Work out the finished part from the listing and answer in its coordinate system (mm). Round coordinates to 2 decimals unless told otherwise and drop trailing zeros. Loops run counter-clockwise (first coordinate to the right, second up) from the corner with the lowest first, then second, coordinate; pieces in that order, holes last. Notation, with made-up numbers: (18, 20) - (69, 20) arc R30 ccw to (69, 43) - close; hole circle Ø1 at (-16, 64). An arc over 180 degrees is marked (long way). Return JSON: item names as keys, results as strings.
from build123d import *

# Parameters (mm, degrees)
SKETCH2_R           = 4
BOSS_EXTRUDE1_DEPTH = 5
FILLET1_R           = 40


with BuildPart() as part:
    # Sketch2 → Boss-Extrude1 (new body)
    with BuildSketch(Plane(origin=(0, -112.700994014, 0), x_dir=(1, 0, 0), z_dir=(0, 1, 0))):
        Polygon((271.436244825, 21.453222376), (186.436244825, 21.453222376), (186.436244825, 274.737493623), (-183.563755175, 274.737493623), (-183.563755175, 21.453222376), (-268.563755175, 21.453222376), (-268.563755175, -91.978235129), (-183.563755175, -91.978235129), (-183.563755175, -345.262506377), (186.436244825, -345.262506377), (186.436244825, -91.978235129), (271.436244825, -91.978235129), align=None)
        with Locations(Location((156.436244825, -325.262506377, 0), (0, 0, 270))):
            Circle(SKETCH2_R, mode=Mode.SUBTRACT)
        with Locations(Location((126.436244825, -325.262506377, 0), (0, 0, 270))):
            Circle(SKETCH2_R, mode=Mode.SUBTRACT)
        with Locations(Location((251.436244825, -61.978235129, 0), (0, 0, 270))):
            Circle(SKETCH2_R, mode=Mode.SUBTRACT)
        with Locations(Location((-153.563755175, -325.262506377, 0), (0, 0, 270))):
            Circle(SKETCH2_R, mode=Mode.SUBTRACT)
        with Locations(Location((-123.563755175, -325.262506377, 0), (0, 0, 270))):
            Circle(SKETCH2_R, mode=Mode.SUBTRACT)
        with Locations(Location((-248.563755175, -61.978235129, 0), (0, 0, 270))):
            Circle(SKETCH2_R, mode=Mode.SUBTRACT)
        with Locations(Location((51.436244825, -275.262506377, 0), (0, 0, 270))):
            Circle(SKETCH2_R, mode=Mode.SUBTRACT)
        with Locations(Location((51.436244825, -65.262506377, 0), (0, 0, 270))):
            Circle(SKETCH2_R, mode=Mode.SUBTRACT)
        with Locations(Location((51.436244825, -5.262506377, 0), (0, 0, 90))):
            Circle(SKETCH2_R, mode=Mode.SUBTRACT)
        with Locations(Location((51.436244825, 204.737493623, 0), (0, 0, 90))):
            Circle(SKETCH2_R, mode=Mode.SUBTRACT)
        with Locations(Location((-248.563755175, -8.546777624, 0), (0, 0, 90))):
            Circle(SKETCH2_R, mode=Mode.SUBTRACT)
        with Locations(Location((-123.563755175, 254.737493623, 0), (0, 0, 90))):
            Circle(SKETCH2_R, mode=Mode.SUBTRACT)
        with Locations(Location((-153.563755175, 254.737493623, 0), (0, 0, 90))):
            Circle(SKETCH2_R, mode=Mode.SUBTRACT)
        with Locations(Location((126.436244825, 254.737493623, 0), (0, 0, 90))):
            Circle(SKETCH2_R, mode=Mode.SUBTRACT)
        with Locations(Location((156.436244825, 254.737493623, 0), (0, 0, 90))):
            Circle(SKETCH2_R, mode=Mode.SUBTRACT)
    extrude(amount=BOSS_EXTRUDE1_DEPTH)

    # Fillet1
    fillet1_edges = [part.edges().sort_by_distance(p)[0] for p in [
        (186.436244825, -110.200994014, -21.453222376),
        (186.436244825, -110.200994014, 91.978235129),
        (-183.563755175, -110.200994014, 91.978235129),
        (-183.563755175, -110.200994014, -21.453222376),
    ]]
    fillet(fillet1_edges, radius=FILLET1_R)


solid = part.part
1) Section A-A (y = -110.6) is taken. Count the separate pieces of the cut face and the enclosed holes in it, and give its area (3 significant figures).
Verdict:
{"separate pieces": "1", "enclosed holes": "15", "area": "249,000 mm2"}
2) Section B-B (z = 164.5) is taken. Give the vertices of the cut face in (x, y).
Verdict:
{"outline": "(-183.56, -112.7) - (186.44, -112.7) - (186.44, -107.7) - (-183.56, -107.7) - close"}
3) Find the intervals of material crossed by L1, parallel to Z at x = -153.5, y = -111.4; L2, parallel to Z at x = 130, y = -109.45; L3, parallel to X at y = -110.25, z = 131.5, in increasing order.
Verdict:
{"L1": "z = -274.74 to -258.74, -250.74 to 321.26, 329.26 to 345.26", "L2": "z = -274.74 to -256.55, -252.92 to 323.45, 327.08 to 345.26", "L3": "x = -183.57 to 186.44"}
4) Flat-ended cylindrical pins translate along their axes: pin 1 (9 mm diameter, centred on x = -153.56, z = -254.74, fed in from -Y); pin 2 (1.5 mm diameter, centred on y = -110, z = -220, fed in from +X); pin 3 (2.5 mm diameter, centred on x = -248, y = -110, fed in from +Z). Find the tip coordinate at first contact, or state that the pin passes through.
Verdict:
{"pin 1": "stops at y = -112.7", "pin 2": "stops at x = 186.44", "pin 3": "stops at z = 91.98"}
5) Section C-C (z = -36) is taken. Give the vertices of the cut face in (x, y).
Verdict:
{"outline": "(-192.71, -112.7) - (195.58, -112.7) - (195.58, -107.7) - (-192.71, -107.7) - close"}
